```python
from build123d import *

# Parameters (mm, degrees)
SKETCH1_W      = 1206.5
SKETCH1_H      = 596.9
EXTRUDE1_DEPTH = 317.5
SKETCH2_W      = 280.957876244
SKETCH2_H      = 93.858968371
EXTRUDE2_DEPTH = 1350.289506876


with BuildPart() as part:
    # Sketch1 → Extrude1 (new body)
    with BuildSketch(Plane(origin=(0, 0, 0), x_dir=(1, 0, 0), z_dir=(0, 1, 0))):
        with Locations((564.434166787, -269.957526684)):
            Rectangle(SKETCH1_W, SKETCH1_H)
    extrude(amount=EXTRUDE1_DEPTH)

    # Sketch2 → Extrude2 (cut, through all)
    with BuildSketch(Plane.XY.offset(568.407526684)):
        with Locations((1027.205228665, 270.570515815)):
            Rectangle(SKETCH2_W, SKETCH2_H)
        with Locations((101.663104909, 270.570515815)):
            Rectangle(SKETCH2_W, SKETCH2_H)
    extrude(amount=-EXTRUDE2_DEPTH, mode=Mode.SUBTRACT)


solid = part.part
```
Read the model definition and answer for the solid it produces. Units are mm, in the model's axes. A direction names the side the tool comes from. Give positions to 0.01 mm unless a question says otherwise; leave off trailing zeros. Loops run counter-clockwise (first coordinate to the right, second up) from the corner with the lowest first, then second, coordinate; pieces in that order, holes last.
Item 1: For faces 1 (the flat face through (886.726, 270, 274)), 2 (the flat face through (556, 121, -28.492)), 3 (the flat face through (100, 223.641, 274)), determine the directions among +Z, -Z, +X, -X, +Y, -Y from which every point of the face is accessible in a straight line to the end or side of a thin tool.
Item 2: The part is cut by section C-C (y = 259). Write down the section's boundary in (x, z), and give its area (3 significant figures).
Item 3: This flat-tipped pin is pushed along its axis until it touches: pin 1 Ø2 at (y, z) = (267, 314) entering from -X. Where does it stop, or does it pass through?
Item 4: The part is cut by section A-A (z = 69). Write down the section's boundary in (x, y).
Item 5: The part is cut by section B-B (x = 902). Write down the section's boundary in (y, z), and give its area (3 significant figures).
Item 6: Find the intervals of material crossed by line 1 along X through (y, z) = (295.5, 228); line 2 along Y through (x, z) = (896, 292), in increasing order.
Taken from the geometry:
1. face 1: +Z, -Z, +X, +Y
1. face 2: -Z, +X, -X, +Y, -Y
1. face 3: +Z, -Z, -X, +Y
2. outline: (242.14, -28.49) - (886.73, -28.49) - (886.73, 568.41) - (242.14, 568.41) - close
2. area: 385,000 mm2
3. pin 1: stops at x = 242.14
4. outline: (-38.82, 0) - (1167.68, 0) - (1167.68, 223.64) - (886.73, 223.64) - (886.73, 317.5) - (242.14, 317.5) - (242.14, 223.64) - (-38.82, 223.64) - close
5. outline: (0, -28.49) - (223.64, -28.49) - (223.64, 568.41) - (0, 568.41) - close
5. area: 133,000 mm2
6. line 1: x = 242.14 to 886.73
6. line 2: y = 0 to 223.64
